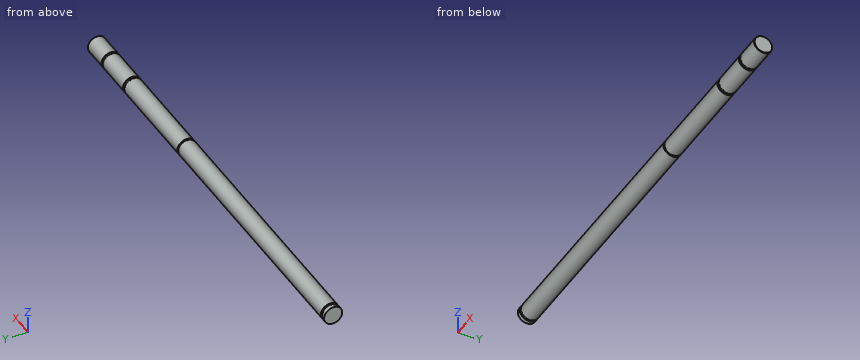
Autodesk Inventor part; units mm, degrees
ref_plane "YZ Plane" through (0, 0, 0) normal (1, 0, 0) x (0, 1, 0)
ref_plane "XZ Plane" through (0, 0, 0) normal (0, 1, 0) x (-1, 0, 0)
ref_plane "XY Plane" through (0, 0, 0) normal (0, 0, 1) x (1, 0, 0)
sketch "Sketch1" plane through (0, 0, 0) normal (0, 0, 1) x (1, 0, 0)
  line L0 (0, 0) -> (0, 5)
  line L1 (0, 5) -> (-14.25, 5)
  line L2 (-14.25, 5) -> (-14.25, 4.5)
  line L3 (-14.25, 4.5) -> (-15.35, 4.5)
  line L4 (-15.35, 4.5) -> (-15.35, 5)
  line L5 (-15.35, 5) -> (-35.85, 5)
  line L6 (-35.85, 5) -> (-35.85, 4.5)
  line L7 (-35.85, 4.5) -> (-36.95, 4.5)
  line L8 (-36.95, 4.5) -> (-36.95, 5)
  line L9 (-235.2, 0) -> (0, 0)
  line L10 (-36.95, 5) -> (-90.4, 5)
  line L11 (-90.4, 5) -> (-90.4, 4.5)
  line L12 (-90.4, 4.5) -> (-91.5, 4.5)
  line L13 (-91.5, 4.5) -> (-91.5, 5)
  line L14 (-91.5, 5) -> (-235.2, 5)
  line L15 (-235.2, 5) -> (-235.2, 4.5)
  line L16 (-235.2, 4.5) -> (-236.3, 4.5)
  line L17 (-236.3, 4.5) -> (-236.3, 5)
  line L18 (-236.3, 5) -> (-238.3, 5)
  line L19 (-238.3, 5) -> (-238.3, 0)
  line L20 (-238.3, 0) -> (-235.2, 0)
  dimension "d0" = 5
  dimension "d1" = 0.5
  dimension "d2" = 1.1
  dimension "d3" = 1.1
  dimension "d4" = 15.35
  dimension "d6" = 35.85
  dimension "d11" = 1.1
  dimension "d12" = 91.5
  dimension "d13" = 1.1
  dimension "d14" = 2
  dimension "d15" = 238.3
revolve "Revolution1" add sketch "Sketch1" angle 360 about axis through (-235.2, 0, 0) along (1, 0, 0)
chamfer "Chamfer1" distance 0.2 angle 45 6 edges at (-235.2, -5, 0) (-35.85, -5, 0) (-36.95, -5, 0) (-14.25, -5, 0) (-15.35, -5, 0) (0, -5, 0)
properties part number "Joint0_LongShaft"
Source: CAD feature listing. Evaluate the final solid. Frame: model axes, mm. Give positions to 0.01 mm unless a question says otherwise; leave off trailing zeros. Loops run counter-clockwise (first coordinate to the right, second up) from the corner with the lowest first, then second, coordinate; pieces in that order, holes last. Notation, with made-up numbers: (82, -36.5) -> (141, -36.5) arc R20 ccw to (141, -22.5) -> close; hole circle Ø10 at (-6, -8.5). An arc over 180 degrees is marked (long way). Use a Markdown table: item, result. Add a question column.
1) Section query A-A, the plane x = -152. Return the cut outline in (y, z).
2) First-contact query: pin 1 (2 mm diameter, centred on x = -152, z = -2, fed in from +Y); pin 2 (4 mm diameter, centred on x = -150, z = 2.5, fed in from +Y); pin 3 (1 mm diameter, centred on x = -200, z = -3.5, fed in from +Y). Flat tips, straight axial feed; report the tip coordinate or a pass-through.
3) Line query: line 1 along X through (y, z) = (-3.25, 3.25); line 2 along Z through (x, y) = (-49, -1.5); line 3 along Z through (x, y) = (-136, -0.5). Output: solid intervals per line, ascending. Write a range as [from, to].
Numbers:
| question | item | result |
|---|---|---|
| 1 | outline | circle Ø10 at (0, 0) |
| 2 | pin 1 | stops at y = 4.9 |
| 2 | pin 2 | stops at y = 4.97 |
| 2 | pin 3 | stops at y = 4 |
| 3 | line 1 | x = [-238.3, -236.3], [-235.2, -91.5], [-90.4, -36.95], [-35.85, -15.35], [-14.25, 0] |
| 3 | line 2 | z = [-4.77, 4.77] |
| 3 | line 3 | z = [-4.97, 4.97] |
